Check sheet for the drawn part. Datum: minimum x, y, z corner. Units: mm. A direction names the side the tool comes from. Coordinates: 2 decimals unless noted, no trailing zeros. Order: outer loops, then holes, each group sorted by start corner. A loop starts at its lowest first (then second) coordinate and runs counter-clockwise, first axis right, second up. Notation, with made-up numbers: M 83,49.5 L 100,49.5 A24 ccw 100,77.5 Z; hole C -33,2.25 d3. An arc over 180 degrees is marked long. Return JSON: item names as keys, results as strings. Group by question number.
Q1. Section check A-A, the plane x = 15. Enter the section's corners in (y, z).
Q2. Access from +Z, -Z, +X, -X, +Y, -Y to the whole of each face (thin tool, end or side, straight path). Record for the marked faces 1 and 2.
Q3. Section check C-C, the plane y = 10. Enter the section's corners in (x, z).
Q4. Mould release check, pull along X, two halves, no side actions. Record for the marked faces 3, 4 and 5: pulls with the +X half, pulls with the -X half, needs draft (parallel to the pull), parting line crosses it, or undercut.
Q5. Go/stop test with flat-tipped pins: pin 1 Ø1 at (y, z) = (3.5, 11) entering from +X; pin 2 Ø6 at (y, z) = (3, 8.5) entering from -X; pin 3 Ø1.6 at (x, z) = (14.5, 11) entering from -Y; pin 4 Ø3.5 at (x, y) = (37.59, 14.75) entering from +Z. Record where each tip stops, or that it passes through.
Q6. Section check D-D, the plane z = 7. Enter the section's corners in (x, y), then the cut area to 3 significant figures.
Q7. Section check B-B, the plane z = 11. Enter the section's corners in (x, y), then the cut area to 3 significant figures.
Q8. Thickness scan on probe 1 along X at (y, z) = (14.75, 7.6); probe 2 along X at (y, z) = (10, 6.75); probe 3 along X at (y, z) = (5.75, 1.25). Record the ranges inside material, lowest first.
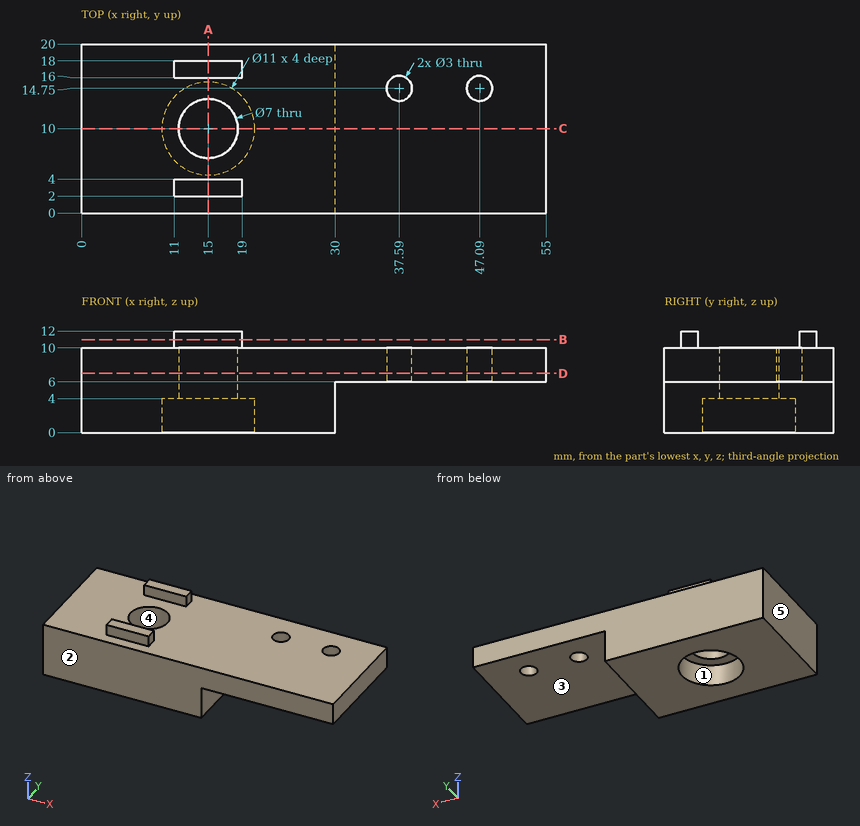
Numbers:
{
 "1": {"outline": "M 0,0 L 4.5,0 L 4.5,4 L 6.5,4 L 6.5,10 L 4,10 L 4,12 L 2,12 L 2,10 L 0,10 Z; M 13.5,4 L 15.5,4 L 15.5,0 L 20,0 L 20,10 L 18,10 L 18,12 L 16,12 L 16,10 L 13.5,10 Z"},
 "2": {"face 1": "-Z", "face 2": "+Z, -Z, +X, -X, -Y"},
 "3": {"outline": "M 0,0 L 9.5,0 L 9.5,4 L 11.5,4 L 11.5,10 L 0,10 Z; M 18.5,4 L 20.5,4 L 20.5,0 L 30,0 L 30,6 L 55,6 L 55,10 L 18.5,10 Z"},
 "4": {"face 3": "needs draft", "face 4": "undercut", "face 5": "pulls with the -X half"},
 "5": {"pin 1": "stops at x = 19", "pin 2": "stops at x = 0", "pin 3": "stops at y = 2", "pin 4": "stops at z = 10"},
 "6": {"outline": "M 0,0 L 55,0 L 55,20 L 0,20 Z; hole C 15,10 d7; hole C 37.59,14.75 d3; hole C 47.09,14.75 d3", "area": "1,050 mm2"},
 "7": {"outline": "M 11,2 L 19,2 L 19,4 L 11,4 Z; M 11,16 L 19,16 L 19,18 L 11,18 Z", "area": "32.0 mm2"},
 "8": {"probe 1": "x = 0 to 36.09, 39.09 to 45.59, 48.59 to 55", "probe 2": "x = 0 to 11.5, 18.5 to 55", "probe 3": "x = 0 to 11.51, 18.49 to 30"}
}
